CAD build for the part. Positions are in the model's coordinates, mm. A direction names the side the tool comes from. Give positions to 0.01 mm unless a question says otherwise; leave off trailing zeros. Loops run counter-clockwise (first coordinate to the right, second up) from the corner with the lowest first, then second, coordinate; pieces in that order, holes last. Notation, with made-up numbers: M 30,15.5 L 80,15.5 A15 ccw 80,23.5 Z; hole C 37,47 d3. An arc over 180 degrees is marked long. One line per question, with ' | ' between items.
```python
from build123d import *

# Parameters (mm, degrees)
SKETCH1_R           = 2.5
BOSS_EXTRUDE1_DEPTH = 3
SKETCH2_R           = 1.4
CUT_EXTRUDE1_DEPTH  = 10


with BuildPart() as part:
    # Sketch1 → Boss-Extrude1 (new, symmetric)
    with BuildSketch(Plane.XY):
        with BuildLine():
            Line((0, 8), (-27, 8))
            ThreePointArc((-27, 8), (-29.121320344, 7.121320344), (-30, 5))
            Line((-30, 5), (-30, 0.1))
            Line((-30, 0.1), (-24.977052658, 3))
            ThreePointArc((-24.977052658, 3), (-14.406610269, -0.585971857), (-4.85358477, -6.359458694))
            ThreePointArc((-4.85358477, -6.359458694), (7.578775282, -2.561672349), (0, 8))
        make_face()
        Circle(SKETCH1_R, mode=Mode.SUBTRACT)
    extrude(amount=BOSS_EXTRUDE1_DEPTH, both=True)

    # Sketch2 → Cut-Extrude1 (cut)
    with BuildSketch(Plane.XY.offset(3)):
        with Locations((-16, 5)):
            Circle(SKETCH2_R)
    extrude(amount=-CUT_EXTRUDE1_DEPTH, mode=Mode.SUBTRACT)


solid = part.part
```
Item 1: Saw through at A-A on y = 0.75. Give the cut face in (x, z).
Conclusion:
outline: M -30,-3 L -28.87,-3 L -28.87,3 L -30,3 Z; M -17.55,-3 L -2.38,-3 L -2.38,3 L -17.55,3 Z; M 2.38,-3 L 7.96,-3 L 7.96,3 L 2.38,3 Z
Item 2: Mould opens along Y. For faces 1 (the cylindrical face through (-29.1, 7.14, 0.04)), 2 (the cylindrical face through (-17.4, 5.06, 0.04)), 3 (the cylindrical face through (-0.54, -2.44, -0.04)), 4 (the cylindrical face through (7.51, -2.76, 0.04)) say: pulls with the +Y half, pulls with the -Y half, needs draft (parallel to the pull), parting line crosses it, or undercut.
Conclusion:
face 1: pulls with the +Y half | face 2: undercut | face 3: undercut | face 4: parting line crosses it
Item 3: Drill centre lines: line 1 along X through (y, z) = (0.5, -1.25); line 2 along X through (y, z) = (4, -1.6); line 3 along X through (y, z) = (-0.5, 1.65). Where is each one in solid material? Low to high. Write a range as [from, to].
Conclusion:
line 1: [-30, -29.31], [-16.91, -2.45], [2.45, 7.98] | line 2: [-30, -16.98], [-15.02, 6.93] | line 3: [-14.59, -2.45], [2.45, 7.98]
Item 4: 3-axis set-ups, long thin cutter, end or side, ignore diameter. For faces 5 (the flat face through (-7, 2, 3)), 6 (the cylindrical face through (-14.55, -0.52, 0.04)): which of +Z, -Z, +X, -X, +Y, -Y reach the whole face in a straight line?
Conclusion:
face 5: +Z, +X, -X, +Y, -Y | face 6: +Z, -Z, -Y
Item 5: Saw through at B-B on z = -0.2. Give the cut face in (x, y), and give its area (3 significant figures).
Conclusion:
outline: M -30,0.1 L -24.98,3 A51.64 cw -4.85,-6.36 A8 ccw long 0,8 L -27,8 A3 ccw -30,5 Z; hole C -16,5 d2.8; hole C 0,0 d5 | area: 357 mm²
Item 6: Drop flat-ended pins along their axis: P1, Ø1, axis at x = -21.5, z = -1, coming from the -Y side; P2, Ø2, axis at x = -19, z = -0.5, coming from the -Y side; P3, Ø1.5, axis at y = -3, z = -2, coming from the +X side. Give the stop position or say it passes through.
Conclusion:
P1: y = 1.95 | P2: y = 0.92 | P3: x = 7.68
Item 7: Saw through at D-D on y = 5.75. Give the cut face in (x, z).
Conclusion:
outline: M -29.9,-3 L -17.18,-3 L -17.18,3 L -29.9,3 Z; M -14.82,-3 L 5.56,-3 L 5.56,3 L -14.82,3 Z
Item 8: Saw through at C-C on x = 0.5. Give the cut face in (y, z), and give its area (3 significant figures).
Conclusion:
outline: M -7.98,-3 L -2.45,-3 L -2.45,3 L -7.98,3 Z; M 2.45,-3 L 7.98,-3 L 7.98,3 L 2.45,3 Z | area: 66.4 mm²
